from build123d import *

# Parameters (mm, degrees)
BOSS_EXTRUDE3_DEPTH = 3
CUT_EXTRUDE2_DEPTH  = 96.033790624


with BuildPart() as part:
    # Sketch1 → Boss-Extrude3 (new body)
    with BuildSketch(Plane(origin=(0, 0, 0), x_dir=(0, 0, -1), z_dir=(1, 0, 0))):
        with BuildLine():
            Line((35.32804493, -2.222841681), (-83.67195507, -2.222841681))
            ThreePointArc((-83.67195507, -2.222841681), (-85.282867773, -6.111928978), (-89.17195507, -7.722841681))
            Line((-89.17195507, -7.722841681), (40.82804493, -7.722841681))
            ThreePointArc((40.82804493, -7.722841681), (36.938957634, -6.111928978), (35.32804493, -2.222841681))
        make_face()
        with BuildLine():
            ThreePointArc((-89.17195507, 3.277158319), (-85.282867773, 1.666245615), (-83.67195507, -2.222841681))
            Line((-83.67195507, -2.222841681), (35.32804493, -2.222841681))
            ThreePointArc((35.32804493, -2.222841681), (36.938957634, 1.666245615), (40.82804493, 3.277158319))
            Line((40.82804493, 3.277158319), (-89.17195507, 3.277158319))
        make_face()
        with BuildLine():
            Line((-89.17195507, -6.072841681), (-89.17195507, -2.222841681))
            Line((-89.17195507, -2.222841681), (-89.17195507, 1.627158319))
            ThreePointArc((-89.17195507, 1.627158319), (-93.02195507, -2.222841681), (-89.17195507, -6.072841681))
        make_face()
        with BuildLine():
            Line((-89.17195507, 1.627158319), (-89.17195507, -2.222841681))
            Line((-89.17195507, -2.222841681), (-85.32195507, -2.222841681))
            ThreePointArc((-85.32195507, -2.222841681), (-86.449593962, 0.499519426), (-89.17195507, 1.627158319))
        make_face()
        with BuildLine():
            Line((-85.32195507, -2.222841681), (-89.17195507, -2.222841681))
            Line((-89.17195507, -2.222841681), (-89.17195507, -6.072841681))
            ThreePointArc((-89.17195507, -6.072841681), (-86.449593962, -4.945202789), (-85.32195507, -2.222841681))
        make_face()
        with BuildLine():
            ThreePointArc((44.67804493, -2.222841681), (43.550406038, 0.499519426), (40.82804493, 1.627158319))
            Line((40.82804493, 1.627158319), (40.82804493, -2.222841681))
            Line((40.82804493, -2.222841681), (40.82804493, -6.072841681))
            ThreePointArc((40.82804493, -6.072841681), (43.550406038, -4.945202789), (44.67804493, -2.222841681))
        make_face()
        with BuildLine():
            ThreePointArc((40.82804493, 1.627158319), (38.105683823, 0.499519426), (36.97804493, -2.222841681))
            Line((36.97804493, -2.222841681), (40.82804493, -2.222841681))
            Line((40.82804493, -2.222841681), (40.82804493, 1.627158319))
        make_face()
        with BuildLine():
            Line((40.82804493, -2.222841681), (36.97804493, -2.222841681))
            ThreePointArc((36.97804493, -2.222841681), (38.105683823, -4.945202789), (40.82804493, -6.072841681))
            Line((40.82804493, -6.072841681), (40.82804493, -2.222841681))
        make_face()
        with BuildLine():
            ThreePointArc((-89.17195507, 1.627158319), (-86.449593962, 0.499519426), (-85.32195507, -2.222841681))
            Line((-85.32195507, -2.222841681), (-83.67195507, -2.222841681))
            ThreePointArc((-83.67195507, -2.222841681), (-85.282867773, 1.666245615), (-89.17195507, 3.277158319))
            Line((-89.17195507, 3.277158319), (-89.17195507, 1.627158319))
        make_face()
        with BuildLine():
            Line((-83.67195507, -2.222841681), (-85.32195507, -2.222841681))
            ThreePointArc((-85.32195507, -2.222841681), (-86.449593962, -4.945202789), (-89.17195507, -6.072841681))
            Line((-89.17195507, -6.072841681), (-89.17195507, -7.722841681))
            ThreePointArc((-89.17195507, -7.722841681), (-85.282867773, -6.111928978), (-83.67195507, -2.222841681))
        make_face()
        with BuildLine():
            ThreePointArc((-89.17195507, -6.072841681), (-93.02195507, -2.222841681), (-89.17195507, 1.627158319))
            Line((-89.17195507, 1.627158319), (-89.17195507, 3.277158319))
            ThreePointArc((-89.17195507, 3.277158319), (-94.67195507, -2.222841681), (-89.17195507, -7.722841681))
            Line((-89.17195507, -7.722841681), (-89.17195507, -6.072841681))
        make_face()
        with BuildLine():
            ThreePointArc((40.82804493, 3.277158319), (36.938957634, 1.666245615), (35.32804493, -2.222841681))
            Line((35.32804493, -2.222841681), (36.97804493, -2.222841681))
            ThreePointArc((36.97804493, -2.222841681), (38.105683823, 0.499519426), (40.82804493, 1.627158319))
            Line((40.82804493, 1.627158319), (40.82804493, 3.277158319))
        make_face()
        with BuildLine():
            Line((36.97804493, -2.222841681), (35.32804493, -2.222841681))
            ThreePointArc((35.32804493, -2.222841681), (36.938957634, -6.111928978), (40.82804493, -7.722841681))
            Line((40.82804493, -7.722841681), (40.82804493, -6.072841681))
            ThreePointArc((40.82804493, -6.072841681), (38.105683823, -4.945202789), (36.97804493, -2.222841681))
        make_face()
        with BuildLine():
            ThreePointArc((46.32804493, -2.222841681), (44.717132227, 1.666245615), (40.82804493, 3.277158319))
            Line((40.82804493, 3.277158319), (40.82804493, 1.627158319))
            ThreePointArc((40.82804493, 1.627158319), (43.550406038, 0.499519426), (44.67804493, -2.222841681))
            ThreePointArc((44.67804493, -2.222841681), (43.550406038, -4.945202789), (40.82804493, -6.072841681))
            Line((40.82804493, -6.072841681), (40.82804493, -7.722841681))
            ThreePointArc((40.82804493, -7.722841681), (44.717132227, -6.111928978), (46.32804493, -2.222841681))
        make_face()
    extrude(amount=BOSS_EXTRUDE3_DEPTH)

    # Sketch1_7 → Cut-Extrude2 (cut, through all)
    with BuildSketch(Plane(origin=(0, 0, 0), x_dir=(0, 0, -1), z_dir=(1, 0, 0))):
        with BuildLine():
            Line((-89.17195507, -6.072841681), (-89.17195507, -2.222841681))
            Line((-89.17195507, -2.222841681), (-89.17195507, 1.627158319))
            ThreePointArc((-89.17195507, 1.627158319), (-93.02195507, -2.222841681), (-89.17195507, -6.072841681))
        make_face()
        with BuildLine():
            Line((-89.17195507, 1.627158319), (-89.17195507, -2.222841681))
            Line((-89.17195507, -2.222841681), (-85.32195507, -2.222841681))
            ThreePointArc((-85.32195507, -2.222841681), (-86.449593962, 0.499519426), (-89.17195507, 1.627158319))
        make_face()
        with BuildLine():
            Line((-85.32195507, -2.222841681), (-89.17195507, -2.222841681))
            Line((-89.17195507, -2.222841681), (-89.17195507, -6.072841681))
            ThreePointArc((-89.17195507, -6.072841681), (-86.449593962, -4.945202789), (-85.32195507, -2.222841681))
        make_face()
        with BuildLine():
            ThreePointArc((44.67804493, -2.222841681), (43.550406038, 0.499519426), (40.82804493, 1.627158319))
            Line((40.82804493, 1.627158319), (40.82804493, -2.222841681))
            Line((40.82804493, -2.222841681), (40.82804493, -6.072841681))
            ThreePointArc((40.82804493, -6.072841681), (43.550406038, -4.945202789), (44.67804493, -2.222841681))
        make_face()
        with BuildLine():
            ThreePointArc((40.82804493, 1.627158319), (38.105683823, 0.499519426), (36.97804493, -2.222841681))
            Line((36.97804493, -2.222841681), (40.82804493, -2.222841681))
            Line((40.82804493, -2.222841681), (40.82804493, 1.627158319))
        make_face()
        with BuildLine():
            Line((40.82804493, -2.222841681), (36.97804493, -2.222841681))
            ThreePointArc((36.97804493, -2.222841681), (38.105683823, -4.945202789), (40.82804493, -6.072841681))
            Line((40.82804493, -6.072841681), (40.82804493, -2.222841681))
        make_face()
    extrude(amount=CUT_EXTRUDE2_DEPTH, mode=Mode.SUBTRACT)


solid = part.part
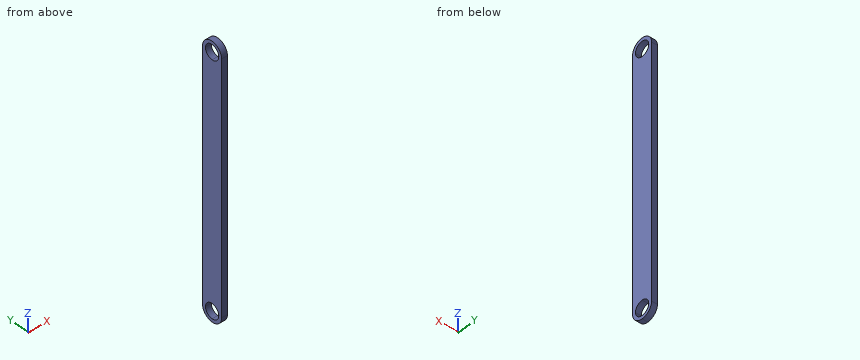
Source: CAD feature listing. Evaluate the final solid. Frame: model axes, mm. Round coordinates to 2 decimals unless told otherwise and drop trailing zeros. Loops run counter-clockwise (first coordinate to the right, second up) from the corner with the lowest first, then second, coordinate; pieces in that order, holes last. Notation, with made-up numbers: (10, 72.5) -> (27, 72.5) arc R25 cw to (27, 103.5) -> close; hole circle Ø9 at (33.5, 72.5). An arc over 180 degrees is marked (long way). Answer as a JSON object with one key per item and string values. Group by question number.
Q1. Ray query, line 1 (Z direction, x = 1.7, y = -2); line 2 (Z direction, x = 2.45, y = -1.5); line 3 (Z direction, x = 1.85, y = -6.25). Return the intervals inside material, ascending. Write a range as from..to.
Q2. Section query A-A (x = 2.4). Output: boundary loops of the cut face in (y, z).
Q3. Section query B-B (y = 0). Output: boundary loops of the cut face in (x, z).
Completed:
{
 "1": {"line 1": "-46.32..-44.67, -36.98..85.33, 93.02..94.67", "line 2": "-46.28..-44.61, -37.05..85.39, 92.95..94.62", "line 3": "-44.57..92.92"},
 "2": {"outline": "(-7.72, -40.83) arc R5.5 ccw to (3.28, -40.83) -> (3.28, 89.17) arc R5.5 ccw to (-7.72, 89.17) -> close; hole circle Ø7.7 at (-2.22, -40.83); hole circle Ø7.7 at (-2.22, 89.17)"},
 "3": {"outline": "(0, -45.86) -> (3, -45.86) -> (3, -43.97) -> (0, -43.97) -> close; (0, -37.68) -> (3, -37.68) -> (3, 86.03) -> (0, 86.03) -> close; (0, 92.32) -> (3, 92.32) -> (3, 94.2) -> (0, 94.2) -> close"}
}
